Source: CAD feature listing. Evaluate the final solid. Frame: model axes, mm. Face numbers are marked on the shaded views. A direction names the side the tool comes from. Give positions to 0.01 mm unless a question says otherwise; leave off trailing zeros. Write each loop counter-clockwise with the first axis right and the second up, starting at its lowest first coordinate (ties: lowest second). Pieces come first, ordered by that corner, then holes. Notation, with made-up numbers: (45.25, 76.25) -> (65.25, 76.25) arc R38 cw to (65.25, 115.25) -> close; hole circle Ø10 at (50.25, 71.25). An arc over 180 degrees is marked (long way). Answer as a JSON object with one key per item and string values. Group by question number.
Item 1: Pull-direction query (X, two-part tool) for the marked faces 1, 2, 3 and 4; classes: pulls with the +X half, pulls with the -X half, needs draft (parallel to the pull), parting line crosses it, or undercut.
Item 2: Section query D-D on y = 36.5. Return the cut outline in (x, z), plus the area to 3 significant figures.
Item 3: Section query B-B on y = 19.5. Return the cut outline in (x, z), plus the area to 3 significant figures.
Item 4: Section query C-C on x = -1. Return the cut outline in (y, z), plus the area to 3 significant figures.
Item 5: Section query A-A on z = -1. Return the cut outline in (x, y).
Item 6: First-contact query: pin 1 Ø1 at (y, z) = (3.5, -2) entering from +X; pin 2 Ø4 at (y, z) = (21, 3) entering from -X; pin 3 Ø1.5 at (x, y) = (-1, 19.5) entering from -Z. Flat tips, straight axial feed; report the tip coordinate or a pass-through.
Item 7: Ray query, probe 1 along X at (y, z) = (1.25, 0); probe 2 along X at (y, z) = (33, 0.25). Return the intervals inside material, ascending. Write a range as from..to.
Item 8: Access query for the marked faces 5 and 6. Directions: +Z, -Z, +X, -X, +Y, -Y. A direction counts if a zero-diameter tool reaches every point of the face in a straight line with its end or side. Return the directions, or none.
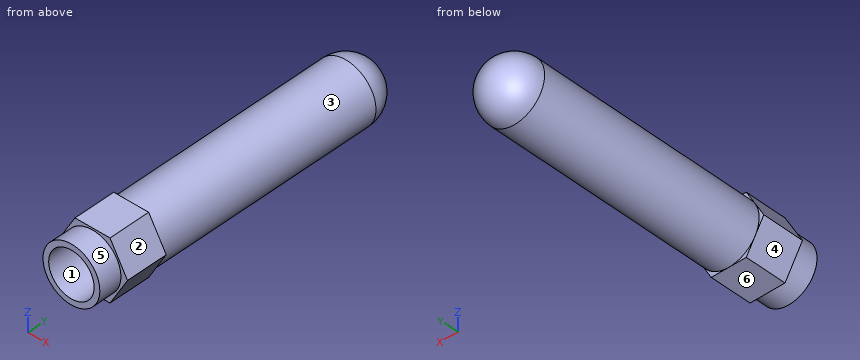
from build123d import *

# Parameters (mm, degrees)
BOSS_EXTRUDE1_DEPTH = 5.5
SKETCH3_R           = 3.75
BOSS_EXTRUDE2_DEPTH = 3
SKETCH4_R           = 3
CUT_EXTRUDE1_DEPTH  = 8


with BuildPart() as part:
    # Sketch1 → Revolve1 (revolve)
    with BuildSketch(Plane.XY):
        with BuildLine():
            Line((0, 0), (4, 0))
            Line((4, 0), (4, 36))
            ThreePointArc((4, 36), (2.828427125, 38.828427125), (0, 40))
            Line((0, 40), (0, 0))
        make_face()
    revolve(axis=Axis((0, 0, 0), (0, 1, 0)))

    # Sketch2 → Boss-Extrude1 (add)
    with BuildSketch(Plane(origin=(0, 0, 0), x_dir=(1, 0, 0), z_dir=(0, 1, 0))):
        Polygon((4.618802154, 0), (2.309401077, 4), (-2.309401077, 4), (-4.618802154, 0), (-2.309401077, -4), (2.309401077, -4), align=None)
    extrude(amount=BOSS_EXTRUDE1_DEPTH)

    # Sketch3 → Boss-Extrude2 (add)
    with BuildSketch(Plane.XZ):
        with Locations(Location((0, 0, 0), (0, 0, 270))):
            Circle(SKETCH3_R)
    extrude(amount=BOSS_EXTRUDE2_DEPTH)

    # Sketch4 → Cut-Extrude1 (cut)
    with BuildSketch(Plane.XZ.offset(3)):
        with Locations(Location((0, 0, 0), (0, 0, 270))):
            Circle(SKETCH4_R)
    extrude(amount=-CUT_EXTRUDE1_DEPTH, mode=Mode.SUBTRACT)


solid = part.part
Worked answers:
{
 "1": {"face 1": "undercut", "face 2": "pulls with the +X half", "face 3": "parting line crosses it", "face 4": "pulls with the -X half"},
 "2": {"outline": "circle Ø7.94 at (0, 0)", "area": "49.5 mm^2"},
 "3": {"outline": "circle Ø8 at (0, 0)", "area": "50.3 mm^2"},
 "4": {"outline": "(-3, -3.61) -> (0, -3.61) -> (0, -4) -> (5.5, -4) -> (5.5, -3.87) -> (36, -3.87) arc R3.87 ccw to (36, 3.87) -> (5.5, 3.87) -> (5.5, 4) -> (0, 4) -> (0, 3.61) -> (-3, 3.61) -> (-3, 2.83) -> (5, 2.83) -> (5, -2.83) -> (-3, -2.83) -> close", "area": "280 mm^2"},
 "5": {"outline": "(-4.04, 0) -> (-3.61, 0) -> (-3.61, -3) -> (-2.83, -3) -> (-2.83, 5) -> (2.83, 5) -> (2.83, -3) -> (3.61, -3) -> (3.61, 0) -> (4.04, 0) -> (4.04, 5.5) -> (3.87, 5.5) -> (3.87, 36) arc R3.87 ccw to (-3.87, 36) -> (-3.87, 5.5) -> (-4.04, 5.5) -> close"},
 "6": {"pin 1": "x = 3.75", "pin 2": "x = -3.87", "pin 3": "z = -3.99"},
 "7": {"probe 1": "-4.62..-3, 3..4.62", "probe 2": "-3.99..3.99"},
 "8": {"face 5": "-Y", "face 6": "-Z, +X, -X, +Y, -Y"}
}
